Geometry: see drawing. Coordinates: mm, zero at the bounding-box minimum. A direction names the side the tool comes from. Coordinates: 2 decimals unless noted, no trailing zeros. Loops run counter-clockwise (first coordinate to the right, second up) from the corner with the lowest first, then second, coordinate; pieces in that order, holes last. Notation, with made-up numbers: (-15.75, -20.75) -> (6.25, -20.75) arc R17 ccw to (6.25, 11.25) -> close; hole circle Ø5 at (-38, 87.25). An arc over 180 degrees is marked (long way). Put each result on its own line as item: value. Start each with the question number.
1) Cut plane A-A (z = 59). Return the cut outline in (x, y) (1 decimal).
2) Cut plane C-C (x = 20). Return the cut outline in (y, z) (1 decimal).
3) Pull-direction query (Z, two-part tool) for the marked faces 1, 2 and 3; classes: pulls with the +Z half, pulls with the -Z half, needs draft (parallel to the pull), parting line crosses it, or undercut.
4) Set-up query: the marked faces 4, 5, 6, 7 and 8. Return all of +Z, -Z, +X, -X, +Y, -Y with unobstructed straight access to the full face (end or side cutting, diameter ignored); none if empty.
5) Cut plane B-B (x = 84). Return the cut outline in (y, z) (1 decimal).
6) Material intervals for L1, parallel to Z at x = 55, y = 17; L2, parallel to Z at x = 20, y = 21 (1 decimal); L3, parallel to Z at x = 87, y = 43 (1 decimal), sorted ascending.
7) Contact query for flat-ended pins moving along their axis: P1, Ø12, axis at y = 22.5, z = 28.5, coming from the +X side (1 decimal); P2, Ø8, axis at y = 19, z = 102, coming from the +X side; P3, Ø1.5, axis at x = 94, z = 57, coming from the +Y side; P4, Ø5, axis at y = 40, z = 95, coming from the +X side. Output: stop coordinate, or through.
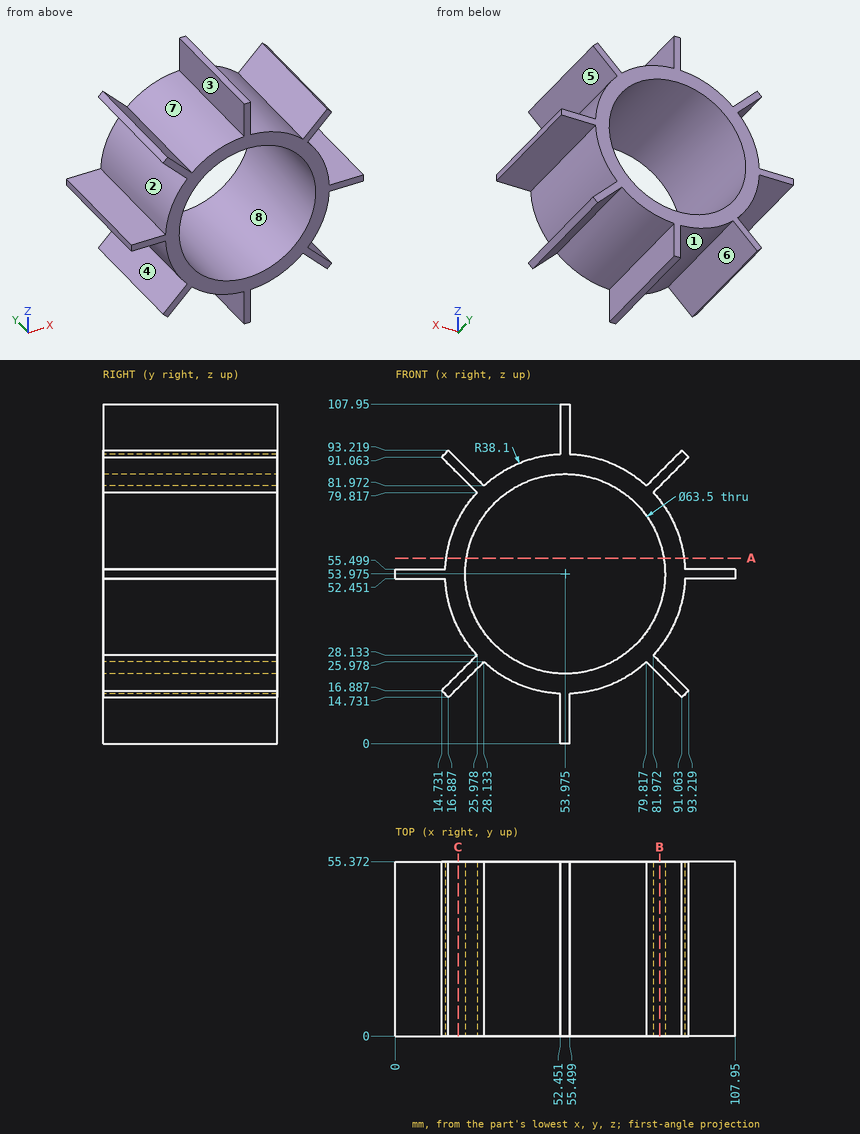
Results found:
1. outline: (16.2, 0) -> (22.6, 0) -> (22.6, 55.4) -> (16.2, 55.4) -> close; (85.3, 0) -> (91.7, 0) -> (91.7, 55.4) -> (85.3, 55.4) -> close
2. outline: (0, 17.8) -> (55.4, 17.8) -> (55.4, 22.2) -> (0, 22.2) -> close; (0, 36.7) -> (55.4, 36.7) -> (55.4, 71.2) -> (0, 71.2) -> close; (0, 85.8) -> (55.4, 85.8) -> (55.4, 90.1) -> (0, 90.1) -> close
3. face 1: pulls with the -Z half
3. face 2: undercut
3. face 3: needs draft
4. face 4: -X, +Y, -Y
4. face 5: +X, +Y, -Y
4. face 6: -Z, +Y, -Y
4. face 7: +Z, +Y, -Y
4. face 8: +Y, -Y
5. outline: (0, 21.8) -> (55.4, 21.8) -> (55.4, 26.1) -> (0, 26.1) -> close; (0, 30.5) -> (55.4, 30.5) -> (55.4, 43.7) -> (0, 43.7) -> close; (0, 64.3) -> (55.4, 64.3) -> (55.4, 77.4) -> (0, 77.4) -> close; (0, 81.8) -> (55.4, 81.8) -> (55.4, 86.2) -> (0, 86.2) -> close
6. L1: z = 0 to 22.24, 85.71 to 107.95
6. L2: z = 17.8 to 22.2, 36.7 to 71.2, 85.8 to 90.1
6. L3: z = 18.8 to 23.1, 35 to 73, 84.8 to 89.2
7. P1: stops at x = 87.6
7. P2: stops at x = 55.5
7. P3: passes through
7. P4: stops at x = 91.78
